Design review of the part built by this model. Coordinates are the model's own, in mm. A direction names the side the tool comes from. Coordinates: 2 decimals unless noted, no trailing zeros. Write each loop counter-clockwise with the first axis right and the second up, starting at its lowest first coordinate (ties: lowest second). Pieces come first, ordered by that corner, then holes. Notation, with made-up numbers: (34.25, 66) -> (76.25, 66) arc R10 ccw to (76.25, 75) -> close; hole circle Ø2 at (6.5, -34). An arc over 180 degrees is marked (long way). Answer in a Markdown table with one row per item. Add a question column.
Item 1: Take a section at B-B, the plane z = -12. Write out the cut boundary in (x, y), and give its area (3 significant figures).
Item 2: To check wall thickness, follow line 1 (X direction, y = 9.15, z = -12); line 2 (Z direction, x = 6.75, y = 1.75); line 3 (X direction, y = 4.25, z = -29). State the ranges of each line that lie inside material, in increasing order.
Item 3: Take a section at C-C, the plane x = 10. Write out the cut boundary in (y, z).
Item 4: Clearance check with flat-ended pins moving along their axes: P1, Ø1.8, axis at x = 4, z = -4.5, coming from the -Y side; P2, Ø4, axis at x = 6, y = 6.5, coming from the +Z side; P3, Ø0.5, axis at x = 12, z = -11.5, coming from the -Y side; P4, Ø1, axis at x = 5.5, z = -25, coming from the +Y side. State where each tip first meets the part, or that it passes through.
Item 5: Take a section at A-A, the plane y = 7.25. Write out the cut boundary in (x, z), and give its area (3 significant figures).
Item 6: Draft analysis for pull direction Z (two halves, no side actions). For faces 1 (the face through (12, 11.2, -28)), 2 (the face through (11.894, 10.389, -17.602)), 3 (the face through (4.78, 8.79, -11.83)), state which applies: released by +Z, released by -Z, zero draft, split by the parting line, or undercut.
Item 7: For faces 4 (the face through (4, 11.2, -20)), 5 (the face through (3.894, 10.389, -17.602)), 6 (the face through (4.306, 8.789, -28.739)), list the 3-axis set-ups (+Z, -Z, +X, -X, +Y, -Y) from which the entire face can be reached by the end or side of a thin tool; tool diameter is ignored.
Item 8: Take a section at D-D, the plane z = -2. Write out the cut boundary in (x, y), and give its area (3 significant figures).
from build123d import *

# Parameters (mm, degrees)
SKETCH1_W            = 16
SKETCH1_H            = 32
BOSS_EXTRUDE1_DEPTH  = 9.6
SKETCH2_R            = 2.4
BOSS_EXTRUDE2_DEPTH  = 1.6
LPATTERN1_COUNT      = 2
LPATTERN1_PITCH      = 8
LPATTERN1_COUNT_DIR2 = 4
LPATTERN1_PITCH_DIR2 = 8
SHELL1_T             = -1.6


with BuildPart() as part:
    # Sketch1 → Boss-Extrude1 (new body)
    with BuildSketch(Plane(origin=(0, 0, 0), x_dir=(1, 0, 0), z_dir=(0, 1, 0))):
        with Locations((8, 16)):
            Rectangle(SKETCH1_W, SKETCH1_H)
    extrude(amount=BOSS_EXTRUDE1_DEPTH)

    # Sketch2 → Boss-Extrude2 (add)
    with BuildSketch(Plane(origin=(0, 9.6, 0), x_dir=(1, 0, 0), z_dir=(0, 1, 0))):
        with Locations(Location((12, 4, 0), (0, 0, 90))):
            Circle(SKETCH2_R)
    boss_extrude2 = extrude(amount=BOSS_EXTRUDE2_DEPTH)

    # LPattern1: Boss-Extrude2 2 × 4
    with Locations(*[(-i * LPATTERN1_PITCH, 0, -j * LPATTERN1_PITCH_DIR2) for i in range(LPATTERN1_COUNT) for j in range(LPATTERN1_COUNT_DIR2) if (i, j) != (0, 0)]):
        add(boss_extrude2)

    # Shell1
    shell1_openings = [part.faces().sort_by_distance(p)[0] for p in [
        (8, 0, -16),
    ]]
    offset(amount=SHELL1_T, openings=shell1_openings, kind=Kind.INTERSECTION)


solid = part.part
Answers:
| question | item | result |
|---|---|---|
| 1 | outline | (0, 0) -> (1.6, 0) -> (1.6, 8) -> (3.2, 8) -> (3.2, 9.6) -> (4.8, 9.6) -> (4.8, 8) -> (11.2, 8) -> (11.2, 9.6) -> (12.8, 9.6) -> (12.8, 8) -> (14.4, 8) -> (14.4, 0) -> (16, 0) -> (16, 9.6) -> (14.4, 9.6) -> (14.4, 11.2) -> (9.6, 11.2) -> (9.6, 9.6) -> (6.4, 9.6) -> (6.4, 11.2) -> (1.6, 11.2) -> (1.6, 9.6) -> (0, 9.6) -> close |
| 1 | area | 61.4 mm^2 |
| 2 | line 1 | x = 0 to 3.2, 4.8 to 11.2, 12.8 to 16 |
| 2 | line 2 | z = -32 to -30.4, -1.6 to 0 |
| 2 | line 3 | x = 0 to 1.6, 14.4 to 16 |
| 3 | outline | (0, -32) -> (9.6, -32) -> (9.6, -29.33) -> (11.2, -29.33) -> (11.2, -26.67) -> (9.6, -26.67) -> (9.6, -21.33) -> (11.2, -21.33) -> (11.2, -18.67) -> (9.6, -18.67) -> (9.6, -13.33) -> (11.2, -13.33) -> (11.2, -10.67) -> (9.6, -10.67) -> (9.6, -5.33) -> (11.2, -5.33) -> (11.2, -2.67) -> (9.6, -2.67) -> (9.6, 0) -> (0, 0) -> (0, -1.6) -> (8, -1.6) -> (8, -30.4) -> (0, -30.4) -> close |
| 4 | P1 | stops at y = 8 |
| 4 | P2 | stops at z = 0 |
| 4 | P3 | stops at y = 9.6 |
| 4 | P4 | stops at y = 9.6 |
| 5 | outline | (0, -32) -> (16, -32) -> (16, 0) -> (0, 0) -> close; hole (1.6, -30.4) -> (14.4, -30.4) -> (14.4, -1.6) -> (1.6, -1.6) -> close |
| 5 | area | 143 mm^2 |
| 6 | face 1 | zero draft |
| 6 | face 2 | undercut |
| 6 | face 3 | undercut |
| 7 | face 4 | +Z, -Z, +X, -X, +Y |
| 7 | face 5 | +Y |
| 7 | face 6 | -Y |
| 8 | outline | (0, 0) -> (1.6, 0) -> (1.6, 8) -> (14.4, 8) -> (14.4, 0) -> (16, 0) -> (16, 9.6) -> (13.33, 9.6) -> (13.33, 11.2) -> (10.67, 11.2) -> (10.67, 9.6) -> (5.33, 9.6) -> (5.33, 11.2) -> (2.67, 11.2) -> (2.67, 9.6) -> (0, 9.6) -> close |
| 8 | area | 59.7 mm^2 |
